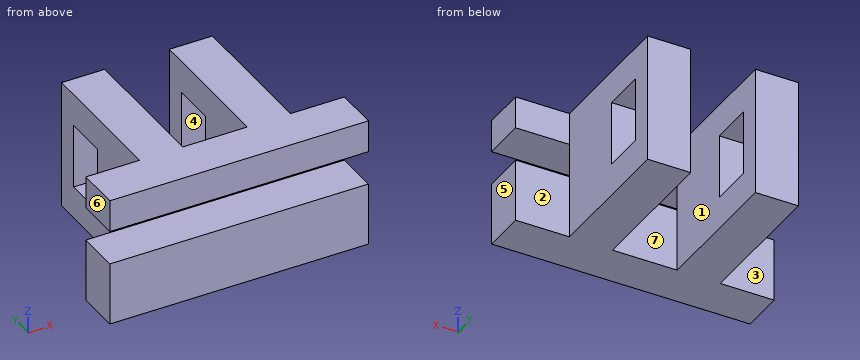
from build123d import *

# Parameters (mm, degrees)
BOSS_EXTRUDE1_DEPTH     = 3
SKETCH4_W               = 12
SKETCH4_H               = 1.5748
CUT_EXTRUDE3_DEPTH      = 2
CUT_EXTRUDE4_DEPTH      = 13.469963913
CUT_EXTRUDE4_DEPTH_BACK = 13.469963913
SKETCH5_W               = 3
SKETCH5_H               = 2


with BuildPart() as part:
    # Sketch1 → Boss-Extrude1 (new, symmetric)
    with BuildSketch(Plane.XY):
        Polygon((-6, -1), (6, -1), (6, 1), (3.5, 1), (3.5, 7.5), (1.5, 7.5), (1.5, 1), (-1.5, 1), (-1.5, 7.5), (-3.5, 7.5), (-3.5, 1), (-6, 1), align=None)
    extrude(amount=BOSS_EXTRUDE1_DEPTH, both=True)

    # Sketch4 → Cut-Extrude3 (cut)
    with BuildSketch(Plane.XZ.offset(1)):
        with Locations((0, 0.7126)):
            Rectangle(SKETCH4_W, SKETCH4_H)
    extrude(amount=-CUT_EXTRUDE3_DEPTH, mode=Mode.SUBTRACT)

    # Sketch5 → Cut-Extrude4 (cut, two sides: drawn at the far end of the back side and taken through both)
    with BuildSketch(Plane.ZY.offset(3.5).offset(-CUT_EXTRUDE4_DEPTH_BACK)):
        with Locations((0, 5.5)):
            Rectangle(SKETCH5_W, SKETCH5_H)
    extrude(amount=CUT_EXTRUDE4_DEPTH + CUT_EXTRUDE4_DEPTH_BACK, mode=Mode.SUBTRACT)


solid = part.part
Build history of the part. All positions in model axes, mm. Face numbers are marked on the shaded views. A direction names the side the tool comes from. Give positions to 0.01 mm unless a question says otherwise; leave off trailing zeros. Loops run counter-clockwise (first coordinate to the right, second up) from the corner with the lowest first, then second, coordinate; pieces in that order, holes last. Notation, with made-up numbers: (58, 51) - (84, 51) arc R27 ccw to (84, 70) - close; hole circle Ø2 at (69.25, -22.75). An arc over 180 degrees is marked (long way). Write item = value, one per line. Start each with the question number.
1) Probe probe 1 along X at (y, z) = (2.5, -1.1); probe 2 along Z at (x, y) = (5.5, 0.75); probe 3 along Z at (x, y) = (2, 6). List the from-to ranges inside material, lowest first. Write a range as from..to.
2) Band-saw the part on C-C on z = -0.4. Give the cut face in (x, y), plus the area to 3 significant figures.
3) Band-saw the part on B-B on x = 1.25. Give the cut face in (y, z), plus the area to 3 significant figures.
4) Band-saw the part on D-D on z = 1.05. Give the cut face in (x, y).
5) Pull direction X, two halves, no side cores. Call the marked faces 5, 6 and 7: +X half, -X half, draft (parallel to the pull), parting line (faces both ways), or undercut.
6) Drop flat-ended pins along their axis: pin 1 Ø3 at (y, z) = (4, -0.5) entering from +X; pin 2 Ø1.6 at (x, z) = (5, 2.5) entering from +Y; pin 3 Ø1.8 at (y, z) = (5.5, -1.5) entering from -X. Give the stop position or say it passes through.
7) Band-saw the part on A-A on y = 6. Give the cut face in (x, z).
8) Tool access for the marked faces 1, 2, 3 and 4: list every direction of +Z, -Z, +X, -X, +Y, -Y with a clear straight run to the whole face (end or side of a thin tool).
Final values:
q1.probe_1 = -3.5..-1.5, 1.5..3.5
q1.probe_2 = -3..-0.07, 1.5..3
q1.probe_3 = -3..-1.5, 1.5..3
q2.outline = (-6, -1) - (6, -1) - (6, 1) - (3.5, 1) - (3.5, 4.5) - (1.5, 4.5) - (1.5, 1) - (-1.5, 1) - (-1.5, 4.5) - (-3.5, 4.5) - (-3.5, 1) - (-6, 1) - close; (-3.5, 6.5) - (-1.5, 6.5) - (-1.5, 7.5) - (-3.5, 7.5) - close; (1.5, 6.5) - (3.5, 6.5) - (3.5, 7.5) - (1.5, 7.5) - close
q2.area = 42.0 mm²
q3.outline = (-1, -3) - (1, -3) - (1, -0.07) - (-1, -0.07) - close; (-1, 1.5) - (1, 1.5) - (1, 3) - (-1, 3) - close
q3.area = 8.85 mm²
q4.outline = (-3.5, 1) - (-1.5, 1) - (-1.5, 4.5) - (-3.5, 4.5) - close; (-3.5, 6.5) - (-1.5, 6.5) - (-1.5, 7.5) - (-3.5, 7.5) - close; (1.5, 1) - (3.5, 1) - (3.5, 4.5) - (1.5, 4.5) - close; (1.5, 6.5) - (3.5, 6.5) - (3.5, 7.5) - (1.5, 7.5) - close
q5.face_5 = +X half
q5.face_6 = -X half
q5.face_7 = undercut
q6.pin_1 = 3.5
q6.pin_2 = 1
q6.pin_3 = -3.5
q7.outline = (-3.5, -3) - (-1.5, -3) - (-1.5, -1.5) - (-3.5, -1.5) - close; (-3.5, 1.5) - (-1.5, 1.5) - (-1.5, 3) - (-3.5, 3) - close; (1.5, -3) - (3.5, -3) - (3.5, -1.5) - (1.5, -1.5) - close; (1.5, 1.5) - (3.5, 1.5) - (3.5, 3) - (1.5, 3) - close
q8.face_1 = +Z, -Z, +Y
q8.face_2 = +Z, -Z, +X, +Y
q8.face_3 = +Z, -Z, -X, +Y
q8.face_4 = +X, -X
